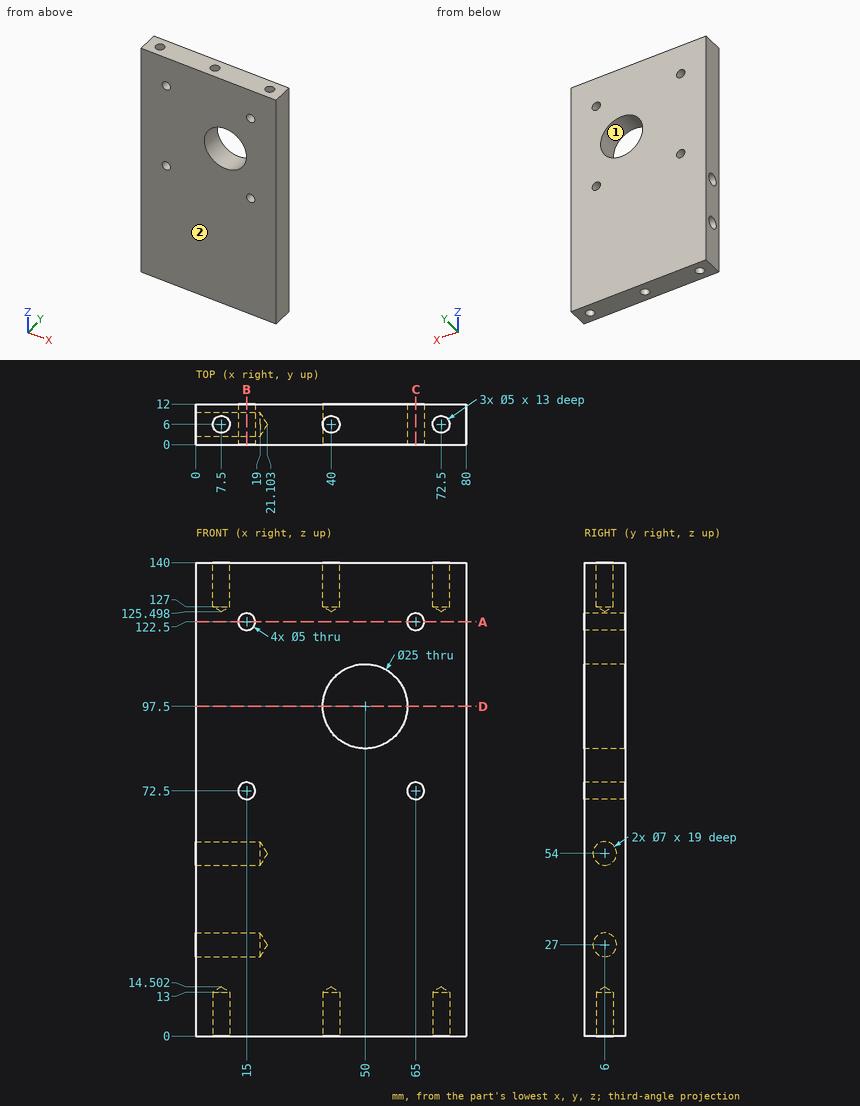
Print and shaded views of the part. All mm, measured from the part's lowest x, y and z. Give positions to 0.01 mm unless a question says otherwise; leave off trailing zeros. Order: outer loops, then holes, each group sorted by start corner. A loop starts at its lowest first (then second) coordinate and runs counter-clockwise, first axis right, second up. Notation, with made-up numbers: M 15,76 L 61,76 A22 ccw 61,111 Z; hole C 32.5,50 d3. An arc over 180 degrees is marked long. Use one line per item in the form item = value.
Q1. Pull direction Z, two halves, no side cores. Call the marked faces 1 and 2: released by +Z, released by -Z, zero draft, split by the parting line, or undercut.
Conclusion:
face_1 = undercut
face_2 = zero draft
Q2. Slice it at A-A, the plane z = 122.5. Write the cut outline in (x, y), and give its area (3 significant figures).
Conclusion:
outline = M 0,0 L 12.5,0 L 12.5,12 L 0,12 Z; M 17.5,0 L 62.5,0 L 62.5,12 L 17.5,12 Z; M 67.5,0 L 80,0 L 80,12 L 67.5,12 Z
area = 840 mm2
Q3. Slice it at C-C, the plane x = 65. Write the cut outline in (y, z), and give its area (3 significant figures).
Conclusion:
outline = M 0,0 L 12,0 L 12,70 L 0,70 Z; M 0,75 L 12,75 L 12,120 L 0,120 Z; M 0,125 L 12,125 L 12,140 L 0,140 Z
area = 1,560 mm2
Q4. Slice it at D-D, the plane z = 97.5. Write the cut outline in (x, y), and give its area (3 significant figures).
Conclusion:
outline = M 0,0 L 37.5,0 L 37.5,12 L 0,12 Z; M 62.5,0 L 80,0 L 80,12 L 62.5,12 Z
area = 660 mm2
Q5. Slice it at B-B, the plane x = 15. Write the cut outline in (y, z), and give its area (3 significant figures).
Conclusion:
outline = M 0,0 L 12,0 L 12,70 L 0,70 Z; M 0,75 L 12,75 L 12,120 L 0,120 Z; M 0,125 L 12,125 L 12,140 L 0,140 Z; hole C 6,27 d7; hole C 6,54 d7
area = 1,480 mm2
Q6. Pin check, flat tips, straight feed: P1, Ø4, axis at x = 7.5, y = 6, coming from the -Z side; P2, Ø5.5, axis at y = 6, z = 54, coming from the -X side; P3, Ø4, axis at x = 72.5, y = 6, coming from the +Z side; P4, Ø4, axis at x = 15, z = 72.5, coming from the +Y side. Stop position of each tip, or through.
Conclusion:
P1 = 13.3
P2 = 19.45
P3 = 126.7
P4 = through
Q7. Wall check: probe 1 along Z at (x, y) = (65, 9.5); probe 2 along X at (y, z) = (6, 133.5); probe 3 along X at (y, z) = (7.75, 72.5). Give the ranges that are in metal, low to high.
Conclusion:
probe_1 = 0 to 70, 75 to 120, 125 to 140
probe_2 = 0 to 5, 10 to 37.5, 42.5 to 70, 75 to 80
probe_3 = 0 to 12.5, 17.5 to 62.5, 67.5 to 80
